Input: part model. Units: mm. Frame: model coordinates. Give positions to 0.01 mm unless a question says otherwise; leave off trailing zeros. Loops run counter-clockwise (first coordinate to the right, second up) from the corner with the lowest first, then second, coordinate; pieces in that order, holes last. Notation, with made-up numbers: (-9, 27) -> (25, 27) arc R25 ccw to (25, 60) -> close; hole circle Ø2 at (58.5, -28). An arc over 180 degrees is marked (long way). Answer as a JSON object with one key per item and string values.
```python
from build123d import *

# Parameters (mm, degrees)
SKETCH1_R           = 1.8
SKETCH1_R_2         = 1.5
SKETCH1_R_3         = 1.35
SKETCH1_R_4         = 44.958
BOSS_EXTRUDE1_DEPTH = 5.842
FILLET1_R           = 4
BOSS_EXTRUDE2_DEPTH = 5.842
FILLET2_R           = 3


with BuildPart() as part:
    # Sketch1 → Boss-Extrude1 (new body)
    # profile 1 of 2: a face of its own
    with BuildSketch(Plane.XY):
        with BuildLine():
            ThreePointArc((50.8, 0), (0, 50.8), (-50.8, 0))
            Line((-50.8, 0), (-50.8, -57.658))
            Line((-50.8, -57.658), (0, -57.658))
            Line((0, -57.658), (50.8, -57.658))
            Line((50.8, -57.658), (50.8, 0))
        make_face()
        with Locations((-41.8, -47.658)):
            Circle(SKETCH1_R, mode=Mode.SUBTRACT)
        with Locations((-33.855565576, -33.855565576)):
            Circle(SKETCH1_R_2, mode=Mode.SUBTRACT)
        with Locations((-41.8, -27.658)):
            Circle(SKETCH1_R, mode=Mode.SUBTRACT)
        with Locations((0, -47.879)):
            Circle(SKETCH1_R_3, mode=Mode.SUBTRACT)
        with Locations((41.8, -47.658)):
            Circle(SKETCH1_R, mode=Mode.SUBTRACT)
        with Locations((33.855565576, -33.855565576)):
            Circle(SKETCH1_R_2, mode=Mode.SUBTRACT)
        with Locations((41.8, -27.658)):
            Circle(SKETCH1_R, mode=Mode.SUBTRACT)
        with Locations((-47.879, 0)):
            Circle(SKETCH1_R_3, mode=Mode.SUBTRACT)
        Circle(SKETCH1_R_4, mode=Mode.SUBTRACT)
        with Locations((-33.855565576, 33.855565576)):
            Circle(SKETCH1_R_2, mode=Mode.SUBTRACT)
        with Locations((0, 47.879)):
            Circle(SKETCH1_R_3, mode=Mode.SUBTRACT)
        with Locations((47.879, 0)):
            Circle(SKETCH1_R_3, mode=Mode.SUBTRACT)
        with Locations((33.855565576, 33.855565576)):
            Circle(SKETCH1_R_2, mode=Mode.SUBTRACT)
    # profile 2 of 2: a face of its own
    with BuildSketch(Plane.XY):
        with BuildLine():
            ThreePointArc((50.8, 0), (0, 50.8), (-50.8, 0))
            Line((-50.8, 0), (-50.8, -57.658))
            Line((-50.8, -57.658), (0, -57.658))
            Line((0, -57.658), (50.8, -57.658))
            Line((50.8, -57.658), (50.8, 0))
        make_face()
        with Locations((-41.8, -47.658)):
            Circle(SKETCH1_R, mode=Mode.SUBTRACT)
        with Locations((-33.855565576, -33.855565576)):
            Circle(SKETCH1_R_2, mode=Mode.SUBTRACT)
        with Locations((-41.8, -27.658)):
            Circle(SKETCH1_R, mode=Mode.SUBTRACT)
        with Locations((0, -47.879)):
            Circle(SKETCH1_R_3, mode=Mode.SUBTRACT)
        with Locations((41.8, -47.658)):
            Circle(SKETCH1_R, mode=Mode.SUBTRACT)
        with Locations((33.855565576, -33.855565576)):
            Circle(SKETCH1_R_2, mode=Mode.SUBTRACT)
        with Locations((41.8, -27.658)):
            Circle(SKETCH1_R, mode=Mode.SUBTRACT)
        with Locations((-47.879, 0)):
            Circle(SKETCH1_R_3, mode=Mode.SUBTRACT)
        Circle(SKETCH1_R_4, mode=Mode.SUBTRACT)
        with Locations((-33.855565576, 33.855565576)):
            Circle(SKETCH1_R_2, mode=Mode.SUBTRACT)
        with Locations((0, 47.879)):
            Circle(SKETCH1_R_3, mode=Mode.SUBTRACT)
        with Locations((47.879, 0)):
            Circle(SKETCH1_R_3, mode=Mode.SUBTRACT)
        with Locations((33.855565576, 33.855565576)):
            Circle(SKETCH1_R_2, mode=Mode.SUBTRACT)
    extrude(amount=BOSS_EXTRUDE1_DEPTH)

    # Fillet1
    fillet1_edges = [part.edges().sort_by_distance(p)[0] for p in [
        (50.8, -57.658, 2.921),
        (-50.8, -57.658, 2.921),
    ]]
    fillet(fillet1_edges, radius=FILLET1_R)

    # Sketch2 → Boss-Extrude2 (add, through all)
    with BuildSketch(Plane.XY.offset(5.842)):
        Polygon((-50.592347052, 4.588509541), (-90.8, 4.588509541), (-90.8, -39.411490459), (-50.8, -39.411490459), align=None)
        with BuildLine():
            Line((-67.8, -33.411490459), (-72.8, -33.411490459))
            ThreePointArc((-72.8, -33.411490459), (-88.8, -17.411490459), (-72.8, -1.411490459))
            Line((-72.8, -1.411490459), (-67.8, -1.411490459))
            ThreePointArc((-67.8, -1.411490459), (-51.8, -17.411490459), (-67.8, -33.411490459))
        make_face(mode=Mode.SUBTRACT)
        with BuildLine():
            Line((-79.8, -1.061490459), (-84.8, -1.061490459))
            ThreePointArc((-84.8, -1.061490459), (-86.45, 0.588509541), (-84.8, 2.238509541))
            Line((-84.8, 2.238509541), (-79.8, 2.238509541))
            ThreePointArc((-79.8, 2.238509541), (-78.15, 0.588509541), (-79.8, -1.061490459))
        make_face(mode=Mode.SUBTRACT)
        with BuildLine():
            Line((-55.8, -1.061490459), (-60.8, -1.061490459))
            ThreePointArc((-60.8, -1.061490459), (-62.45, 0.588509541), (-60.8, 2.238509541))
            Line((-60.8, 2.238509541), (-55.8, 2.238509541))
            ThreePointArc((-55.8, 2.238509541), (-54.15, 0.588509541), (-55.8, -1.061490459))
        make_face(mode=Mode.SUBTRACT)
        with BuildLine():
            Line((-79.8, -37.061490459), (-84.8, -37.061490459))
            ThreePointArc((-84.8, -37.061490459), (-86.45, -35.411490459), (-84.8, -33.761490459))
            Line((-84.8, -33.761490459), (-79.8, -33.761490459))
            ThreePointArc((-79.8, -33.761490459), (-78.15, -35.411490459), (-79.8, -37.061490459))
        make_face(mode=Mode.SUBTRACT)
        with BuildLine():
            Line((-55.8, -37.061490459), (-60.8, -37.061490459))
            ThreePointArc((-60.8, -37.061490459), (-62.45, -35.411490459), (-60.8, -33.761490459))
            Line((-60.8, -33.761490459), (-55.8, -33.761490459))
            ThreePointArc((-55.8, -33.761490459), (-54.15, -35.411490459), (-55.8, -37.061490459))
        make_face(mode=Mode.SUBTRACT)
    extrude(amount=-BOSS_EXTRUDE2_DEPTH)

    # Fillet2
    fillet2_edges = [part.edges().sort_by_distance(p)[0] for p in [
        (-50.8, -39.411490459, 2.921),
        (-90.8, -39.411490459, 2.921),
        (-90.8, 4.588509541, 2.921),
    ]]
    fillet(fillet2_edges, radius=FILLET2_R)


solid = part.part
```
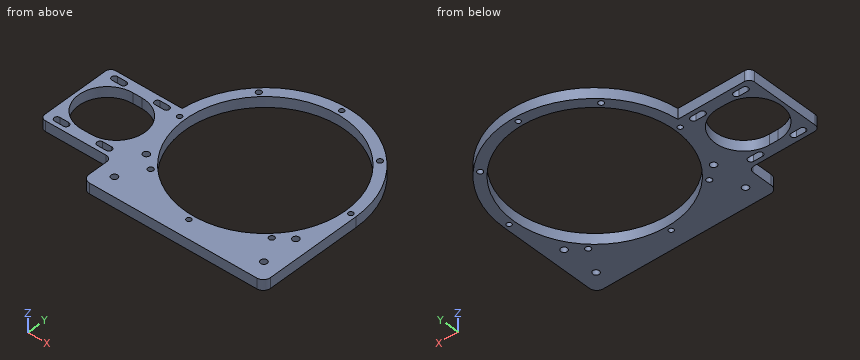
Q1. Section D-D, the plane z = 2.6. Give the number of separate pieces and of enclosed holes in the cut face, then the cut area to 3 significant figures.
Evaluation:
{"separate pieces": "1", "enclosed holes": "18", "area": "4,160 mm2"}
Q2. Ray query, line 1 along Y through (x, z) = (0, 1.95); line 2 along X through (y, z) = (-11, 2.9); line 3 along Y through (x, z) = (-1.5, 3.05). Return the intervals inside material, ascending.
Evaluation:
{"line 1": "y = -57.66 to -49.23, -46.53 to -44.96, 44.96 to 46.53, 49.23 to 50.8", "line 2": "x = -90.8 to -87.46, -53.14 to -43.59, 43.59 to 50.8", "line 3": "y = -57.66 to -44.93, 44.93 to 50.78"}
Q3. Section B-B, the plane y = 14. Return the cut outline in (x, z).
Evaluation:
{"outline": "(-48.83, 0) -> (-42.72, 0) -> (-42.72, 5.84) -> (-48.83, 5.84) -> close; (42.72, 0) -> (48.83, 0) -> (48.83, 5.84) -> (42.72, 5.84) -> close"}
Q4. Section A-A, the plane x = -4. Return the cut outline in (y, z), then the cut area to 3 significant figures.
Evaluation:
{"outline": "(-57.66, 0) -> (-44.78, 0) -> (-44.78, 5.84) -> (-57.66, 5.84) -> close; (44.78, 0) -> (50.64, 0) -> (50.64, 5.84) -> (44.78, 5.84) -> close", "area": "109 mm2"}
Q5. Section C-C, the plane x = -41.8. Return the cut outline in (y, z), then the cut area to 3 significant figures.
Evaluation:
{"outline": "(-57.66, 0) -> (-49.46, 0) -> (-49.46, 5.84) -> (-57.66, 5.84) -> close; (-45.86, 0) -> (-29.46, 0) -> (-29.46, 5.84) -> (-45.86, 5.84) -> close; (-25.86, 0) -> (-16.55, 0) -> (-16.55, 5.84) -> (-25.86, 5.84) -> close; (16.55, 0) -> (28.87, 0) -> (28.87, 5.84) -> (16.55, 5.84) -> close", "area": "270 mm2"}
Q6. Pin query (flat end, axial travel): pin 1 (2.5 mm diameter, centred on x = -83, z = 3.5, fed in from -Y); pin 2 (3 mm diameter, centred on y = -48, z = 2.5, fed in from -X). Return the tip coordinate at first contact, or that it passes through.
Evaluation:
{"pin 1": "stops at y = -39.41", "pin 2": "stops at x = -50.8"}
